Can you work these out from the model? Positions are in its coordinate system, mm. A direction names the side the tool comes from. Round coordinates to 2 decimals unless told otherwise and drop trailing zeros. Write each loop counter-clockwise with the first axis right and the second up, starting at its lowest first coordinate (ties: lowest second). Pieces come first, ordered by that corner, then holes. Notation, with made-up numbers: (-10, 19.25) -> (32, 19.25) arc R9 ccw to (32, 25.25) -> close; hole circle Ø5 at (28, 58). An arc over 180 degrees is marked (long way). Use CSV: the item, a comma, the result in double quotes.
```python
from build123d import *

# Parameters (mm, degrees)
SKETCH1_R           = 15
SKETCH1_R_2         = 12.5
BOSS_EXTRUDE1_DEPTH = 25
BOSS_EXTRUDE2_START = 20
SKETCH1_2_R         = 12.5
BOSS_EXTRUDE2_DEPTH = 5
BOSS_EXTRUDE3_START = -20
SKETCH1_3_R         = 12.5
BOSS_EXTRUDE3_DEPTH = 5
SKETCH2_R           = 2.5
CUT_EXTRUDE1_DEPTH  = 16


with BuildPart() as part:
    # Sketch1 → Boss-Extrude1 (new body, symmetric)
    with BuildSketch(Plane(origin=(0, 0, 0), x_dir=(0, 0, -1), z_dir=(1, 0, 0))):
        Circle(SKETCH1_R)
        Circle(SKETCH1_R_2, mode=Mode.SUBTRACT)
    extrude(amount=BOSS_EXTRUDE1_DEPTH, both=True)

    # Sketch1_2 → Boss-Extrude2 (add)
    with BuildSketch(Plane(origin=(0, 0, 0), x_dir=(0, 0, -1), z_dir=(1, 0, 0)).offset(BOSS_EXTRUDE2_START)):
        Circle(SKETCH1_2_R)
    extrude(amount=BOSS_EXTRUDE2_DEPTH)

    # Sketch1_3 → Boss-Extrude3 (add)
    with BuildSketch(Plane(origin=(0, 0, 0), x_dir=(0, 0, -1), z_dir=(1, 0, 0)).offset(BOSS_EXTRUDE3_START)):
        Circle(SKETCH1_3_R)
    extrude(amount=-BOSS_EXTRUDE3_DEPTH)

    # Sketch2 → Cut-Extrude1 (cut, through all)
    with BuildSketch(Plane(origin=(0, 0, 0), x_dir=(1, 0, 0), z_dir=(0, 1, 0))):
        with Locations((-15, 0)):
            Circle(SKETCH2_R)
        with Locations((15, 0)):
            Circle(SKETCH2_R)
    extrude(amount=CUT_EXTRUDE1_DEPTH, mode=Mode.SUBTRACT)


solid = part.part
```
Q1. Will these pins go through, and if not, where does the flat tip stop? P1, Ø2, axis at x = -11.5, z = 2.5, coming from the -Y side; P2, Ø3, axis at x = -15, z = 0, coming from the +Y side; P3, Ø1.5, axis at x = -10, y = 5, coming from the +Z side.
Resolved:
P1,"stops at y = -14.92"
P2,"stops at y = -12.41"
P3,"stops at z = 14.39"
Q2. Suppose I cut it at B-B (y = 0). Write out the boundary of the cut face in (x, z).
Resolved:
outline,"(-25, -15) -> (25, -15) -> (25, 15) -> (-25, 15) -> close; hole (-20, -12.5) -> (20, -12.5) -> (20, 12.5) -> (-20, 12.5) -> close"
Q3. On a 3-axis mill with a long thin cutter (end or side, diameter ignored), from which of +Z, -Z, +X, -X, +Y, -Y can I reach the whole of each face in a straight line? I mean faces 1 (the face through (-20, 0, 0)), 2 (the face through (0.35, -14.643, 3.252)). Say none if no direction works.
Resolved:
face 1,"none"
face 2,"+X, -X"
Q4. Please list where these lines run through material, in increasing order: probe 1 along X at (y, z) = (12.95, 0); probe 2 along X at (y, z) = (-5.5, 8.5); probe 3 along Y at (x, z) = (18, -11).
Resolved:
probe 1,"x = -25 to -17.5, -12.5 to 12.5, 17.5 to 25"
probe 2,"x = -25 to -20, 20 to 25"
probe 3,"y = -10.2 to -5.94, 5.94 to 10.2"
Q5. Suppose I cut it at D-D (x = -9.5). Write out the boundary of the cut face in (y, z), and give its area (3 significant figures).
Resolved:
outline,"circle Ø30 at (0, 0); hole circle Ø25 at (0, 0)"
area,"216 mm^2"
Q6. If we mould it in two halves opening along X, with no side actions, what happens to faces 3 (the face through (17.31, 13.61, 0.96)), 4 (the face through (-25, 0, 0)), 5 (the face through (25, 0, 0)), 6 (the face through (-12.615, 13.607, -0.751))? For each: released by +X, released by -X, zero draft, split by the parting line, or undercut.
Resolved:
face 3,"undercut"
face 4,"released by -X"
face 5,"released by +X"
face 6,"undercut"
Q7. Suppose I cut it at A-A (z = 0). Write out the boundary of the cut face in (x, y).
Resolved:
outline,"(-25, -15) -> (25, -15) -> (25, 15) -> (17.5, 15) -> (17.5, 12.5) -> (20, 12.5) -> (20, -12.5) -> (-20, -12.5) -> (-20, 12.5) -> (-17.5, 12.5) -> (-17.5, 15) -> (-25, 15) -> close; (-12.5, 12.5) -> (12.5, 12.5) -> (12.5, 15) -> (-12.5, 15) -> close"
Q8. Suppose I cut it at C-C (z = 4). Write out the boundary of the cut face in (x, y), and give its area (3 significant figures).
Resolved:
outline,"(-25, -14.46) -> (25, -14.46) -> (25, 14.46) -> (-25, 14.46) -> close; hole (-20, -11.84) -> (20, -11.84) -> (20, 11.84) -> (-20, 11.84) -> close"
area,"498 mm^2"
